Autodesk Inventor part; units mm, degrees
ref_plane "YZ Plane" through (0, 0, 0) normal (1, 0, 0) x (0, 1, 0)
ref_plane "XZ Plane" through (0, 0, 0) normal (0, 1, 0) x (-1, 0, 0)
ref_plane "XY Plane" through (0, 0, 0) normal (0, 0, 1) x (1, 0, 0)
sketch "Esquisse1" plane through (0, 0, 0) normal (0, 0, 1) x (1, 0, 0)
  circle A0 centre (0, 0) radius 13.5
  circle A1 centre (0, 0) radius 8.25
  dimension "d0" = 27
  dimension "d1" = 16.5
extrude "Extrusion1" add sketch "Esquisse1" along normal blind 23.5
sketch "Esquisse2" plane through (0, 0, 23.5) normal (0, 0, 1) x (1, 0, 0)
  circle A0 centre (0, 0) radius 8.25
extrude "Extrusion2" add sketch "Esquisse2" against normal blind 1.3
sketch "Esquisse3" plane through (0, 0, 0) normal (0, 0, -1) x (-1, 0, 0)
  line L0 (-2.1903, 13.3211) -> (-2.1903, 11.85)
  line L1 (-2.1903, 11.85) -> (0, 11.85)
  line L2 (0, 11.85) -> (2.1903, 11.85)
  line L3 (2.1903, 13.3211) -> (2.1903, 11.85)
  arc A0 (0, 13.5) -> (-2.1903, 13.3211) centre (0, 0) ccw
  arc A1 (2.1903, 13.3211) -> (0, 13.5) centre (0, 0) ccw
  arc A2 (0, -13.5) -> (2.1903, -13.3211) centre (0, 0) ccw
  arc A3 (-2.1903, -13.3211) -> (0, -13.5) centre (0, 0) ccw
  line L4 (-2.1903, -13.3211) -> (-2.1903, -11.85)
  line L5 (0, -11.85) -> (-2.1903, -11.85)
  line L6 (2.1903, -11.85) -> (0, -11.85)
  line L7 (2.1903, -13.3211) -> (2.1903, -11.85)
  point P0 (0, 0)
  point P1 (0, -50)
  point P2 (-13.5, 0)
extrude "Extrusion3" cut sketch "Esquisse3" against normal blind 2.5
sketch "Esquisse4" plane through (0, 0, 23.5) normal (0, 0, 1) x (1, 0, 0)
  line L0 (-2.1903, 13.3211) -> (-2.1903, 11.85)
  line L1 (-2.1903, 11.85) -> (0, 11.85)
  line L2 (0, 11.85) -> (2.1903, 11.85)
  line L3 (2.1903, 13.3211) -> (2.1903, 11.85)
  arc A0 (0, 13.5) -> (-2.1903, 13.3211) centre (0, 0) ccw
  arc A1 (2.1903, 13.3211) -> (0, 13.5) centre (0, 0) ccw
  arc A2 (0, -13.5) -> (2.1903, -13.3211) centre (0, 0) ccw
  arc A3 (-2.1903, -13.3211) -> (0, -13.5) centre (0, 0) ccw
  line L4 (-2.1903, -13.3211) -> (-2.1903, -11.85)
  line L5 (0, -11.85) -> (-2.1903, -11.85)
  line L6 (2.1903, -11.85) -> (0, -11.85)
  line L7 (2.1903, -13.3211) -> (2.1903, -11.85)
  point P0 (0, 0)
  point P1 (0, 0)
extrude "Extrusion4" cut sketch "Esquisse4" against normal blind 2.5
properties part number "pièce intermédiaire"
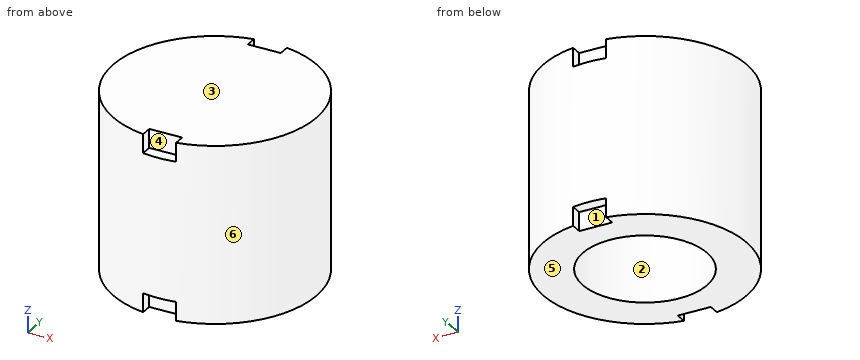
Geometry check sheet. Reference: the model listing, model coordinates, mm. Face numbers are marked on the shaded views. A direction names the side the tool comes from. Round coordinates to 2 decimals unless told otherwise and drop trailing zeros. Order: outer loops, then holes, each group sorted by start corner. A loop starts at its lowest first (then second) coordinate and runs counter-clockwise, first axis right, second up. Notation, with made-up numbers: M 10,-36.75 L 18,-36.75 A21 cw 18,-1.75 Z; hole C 14,67.5 d10. An arc over 180 degrees is marked long. Answer as CSV lines item,"result".
1) Sectioned sample at C-C on y = 0. Record the cut outline in (x, z), and give its area (3 significant figures).
Entries:
outline,"M -13.5,0 L -8.25,0 L -8.25,22.2 L 8.25,22.2 L 8.25,0 L 13.5,0 L 13.5,23.5 L -13.5,23.5 Z"
area,"268 mm2"
2) Sectioned sample at A-A on z = 1.75. Record the cut outline in (x, y), and give its area (3 significant figures).
Entries:
outline,"M -2.19,-13.32 L -2.19,-11.85 L 2.19,-11.85 L 2.19,-13.32 A13.5 ccw 2.19,13.32 L 2.19,11.85 L -2.19,11.85 L -2.19,13.32 A13.5 ccw Z; hole C 0,0 d16.5"
area,"345 mm2"
3) Sectioned sample at D-D on x = 5. Record the cut outline in (y, z), and give its area (3 significant figures).
Entries:
outline,"M -12.54,0 L -6.56,0 L -6.56,22.2 L 6.56,22.2 L 6.56,0 L 12.54,0 L 12.54,23.5 L -12.54,23.5 Z"
area,"298 mm2"
4) Sectioned sample at B-B on x = 0. Record the cut outline in (y, z).
Entries:
outline,"M -13.5,2.5 L -11.85,2.5 L -11.85,0 L -8.25,0 L -8.25,22.2 L 8.25,22.2 L 8.25,0 L 11.85,0 L 11.85,2.5 L 13.5,2.5 L 13.5,21 L 11.85,21 L 11.85,23.5 L -11.85,23.5 L -11.85,21 L -13.5,21 Z"
5) Tool access check on the marked faces 1, 2 and 3. Record the directions out of +Z, -Z, +X, -X, +Y, -Y that give a thin tool (end or side, any length) a straight path to the whole face; none if there is none.
Entries:
face 1,"-Z, +Y"
face 2,"-Z"
face 3,"+Z, +X, -X, +Y, -Y"
6) Thickness scan on probe 1 along Y at (x, z) = (0, 13.5); probe 2 along Y at (x, z) = (-7, 1.75); probe 3 along X at (y, z) = (5.5, 18.25). Record the ranges inside material, lowest first. Write a range as [from, to].
Entries:
probe 1,"[-13.5, -8.25], [8.25, 13.5]"
probe 2,"[-11.54, -4.37], [4.37, 11.54]"
probe 3,"[-12.33, -6.15], [6.15, 12.33]"
7) Gauge pin test, flat ends, axial feed: pin 1 Ø1.2 at (y, z) = (-13, 1) entering from -X; pin 2 Ø1.2 at (x, z) = (-0.5, 1) entering from +Y; pin 3 Ø3 at (x, z) = (-8.5, 15.5) entering from +Y. Record the tip position at first contact, or that the pin passes through.
Entries:
pin 1,"x = -5.34"
pin 2,"y = 11.85"
pin 3,"y = 11.54"
8) Mould release check, pull along X, two halves, no side actions. Record for the marked faces 4, 5 and 6: +X half, -X half, draft (parallel to the pull), parting line (faces both ways), or undercut.
Entries:
face 4,"undercut"
face 5,"draft"
face 6,"parting line"
